from build123d import *

# Parameters (mm, degrees)
SKETCH037_R          = 1.6
SKETCH037_R_2        = 17
PAD006_DEPTH         = 3
SKETCH003_R          = 1.5
PAD007_DEPTH         = 22
SKETCH042_R          = 33.309059
POCKET028_DEPTH      = 18.95
SKETCH043_W          = 51.697506
SKETCH043_H          = 15.935999
POCKET029_DEPTH      = 28.801
POCKET029_DEPTH_BACK = 23.4566344398
SKETCH040_R          = 3
FILLET003_R          = 2
FILLET004_R          = 5
FILLET005_R          = 1


with BuildPart() as part:
    # Sketch037 → Pad006 (new body)
    with BuildSketch(Plane.XY.offset(8)):
        with BuildLine():
            Line((-25.5, 14.6837073124), (-25.5, -7.8162926876))
            Line((-5.3310209809, -19.2403151033), (-25.5, -7.8162926876))
            Line((11.1640063658, -23.3529873285), (-5.3310209809, -19.2403151033))
            ThreePointArc((11.1640063658, -23.3529873285), (13.7797833094, -22.9620568449), (15.3529873285, -20.8359936342))
            Line((19.8, -3), (15.3529873285, -20.8359936342))
            Line((19.8, 15.1005154776), (19.8, -3))
            ThreePointArc((19.8, 15.1005154776), (19.1301270189, 17.6005154776), (17.3, 19.4306424965))
            Line((2, 28.2641016151), (17.3, 19.4306424965))
            ThreePointArc((2, 28.2641016151), (0, 28.8), (-2, 28.2641016151))
            Line((-9.101080859, 23.5924155561), (-2, 28.2641016151))
            ThreePointArc((-15.8499401029, 19.751877), (-10.97303678, 19.0318958608), (-9.101080859, 23.5924155561))
            Line((-25.5, 14.6837073124), (-15.8499401029, 19.751877))
        make_face()
        with Locations((0, 24.8)):
            Circle(SKETCH037_R, mode=Mode.SUBTRACT)
        with Locations((12, -20)):
            Circle(SKETCH037_R, mode=Mode.SUBTRACT)
        with Locations((-21.5, 12.3)):
            Circle(SKETCH037_R, mode=Mode.SUBTRACT)
        Circle(SKETCH037_R_2, mode=Mode.SUBTRACT)
    extrude(amount=PAD006_DEPTH)

    # Sketch003 → Pad007 (join)
    with BuildSketch(Plane(origin=(-2.6, 10.8, 17), x_dir=(0.9021044144, 0.420580995, -0.0965362737), z_dir=(-0.1354559934, 0.4884043208, 0.8620399604))):
        with BuildLine():
            Line((-23.3696005315, -4.8773641565), (-13.621692219, 4.2127074032))
            ThreePointArc((-12.2576954989, 4.75), (-12.9906979524, 4.610835136), (-13.621692219, 4.2127074032))
            Line((-12.2576954989, 4.75), (10.0610339657, 4.75))
            ThreePointArc((10.780373766, 4.4446583705), (10.4517650942, 4.6705048535), (10.0610339657, 4.75))
            Line((10.780373766, 4.4446583705), (19.7793336026, -4.8740373329))
            ThreePointArc((21.0423045011, -8), (20.7146318466, -6.3142703296), (19.7793336026, -4.8740373329))
            Line((21.0423045011, -8), (21.0423045011, -15.35))
            ThreePointArc((20.0423045011, -16.35), (20.7494112823, -16.0571067812), (21.0423045011, -15.35))
            Line((20.0423045011, -16.35), (-8.9576954989, -16.35))
            Line((-8.9576954989, -16.35), (-21.8124305048, -12.0490416884))
            ThreePointArc((-23.3696005315, -4.8773641565), (-24.6301401013, -8.9059534041), (-21.8124305048, -12.0490416884))
        make_face()
        with Locations((16.5423045011, -8)):
            Circle(SKETCH003_R, mode=Mode.SUBTRACT)
        with Locations((-20.4576954989, -8)):
            Circle(SKETCH003_R, mode=Mode.SUBTRACT)
    extrude(amount=-PAD007_DEPTH)

    # Sketch042 → Pocket028 (cut, symmetric)
    with BuildSketch(Plane.XY.offset(8)):
        with Locations((0, 3.706026)):
            Circle(SKETCH042_R)
        with BuildLine():
            Line((-25.5, 14.6963702892), (-25.5, -7.8036297108))
            Line((-5.3310209809, -19.2403151033), (-25.5, -7.8036297108))
            Line((11.1640063658, -23.3529873285), (-5.3310209809, -19.2403151033))
            ThreePointArc((11.1640063658, -23.3529873285), (13.7797833094, -22.9620568449), (15.3529873285, -20.8359936342))
            Line((19.8, -3), (15.3529873285, -20.8359936342))
            Line((19.8, 15.1005154776), (19.8, -3))
            ThreePointArc((19.8, 15.1005154776), (19.1301270189, 17.6005154776), (17.3, 19.4306424965))
            Line((2, 28.2641016151), (17.3, 19.4306424965))
            ThreePointArc((2, 28.2641016151), (0, 28.8), (-2, 28.2641016151))
            Line((-25.5, 14.6963702892), (-2, 28.2641016151))
        make_face(mode=Mode.SUBTRACT)
    extrude(amount=POCKET028_DEPTH, both=True, mode=Mode.SUBTRACT)

    # Sketch043 → Pocket029 (cut, two sides)
    with BuildSketch(Plane.XZ) as pocket029_sk:
        with Locations((-1.406603, 0.0320005)):
            Rectangle(SKETCH043_W, SKETCH043_H)
    extrude(amount=-POCKET029_DEPTH, mode=Mode.SUBTRACT)
    extrude(pocket029_sk.sketch, amount=POCKET029_DEPTH_BACK, mode=Mode.SUBTRACT)

    # SubtractivePipe: sweep along a path in Sketch044
    with BuildLine(Plane(origin=(0, 0, 6), x_dir=(-0.3746065934, 0.9271838546, 0), z_dir=(0.9266190392, 0.3743783932, 0.0348994967))) as subtractivepipe_path:
        ThreePointArc((4.9840972168, 16.8364980654), (1.2784963095, 9.7214039712), (0, 1.801714))
    # Sketch040 → SubtractivePipe (sweep, cut)
    with BuildSketch(Plane(origin=(-2, 7.6, 8), x_dir=(0.8829475929, 0.4694715628, 0), z_dir=(0, 0, 1))):
        with Locations((-1.846382, -7.651343)):
            Circle(SKETCH040_R)
    sweep(path=subtractivepipe_path.line, mode=Mode.SUBTRACT)

    # Fillet003
    fillet003_edges = [part.edges().sort_by_distance(p)[0] for p in [
        (-9.101081, 23.592416, 9.5),
        (-15.84994, 19.751877, 9.5),
    ]]
    fillet(fillet003_edges, radius=FILLET003_R)

    # Fillet004
    fillet004_edges = [part.edges().sort_by_distance(p)[0] for p in [
        (-25.5, -7.80363, 9.5),
        (-25.5, 14.683707, 9.5),
    ]]
    fillet(fillet004_edges, radius=FILLET004_R)

    # Fillet005
    fillet005_edges = [part.edges().sort_by_distance(p)[0] for p in [
        (-4.660699, 2.190867, 21.553854),
    ]]
    fillet(fillet005_edges, radius=FILLET005_R)


solid = part.part
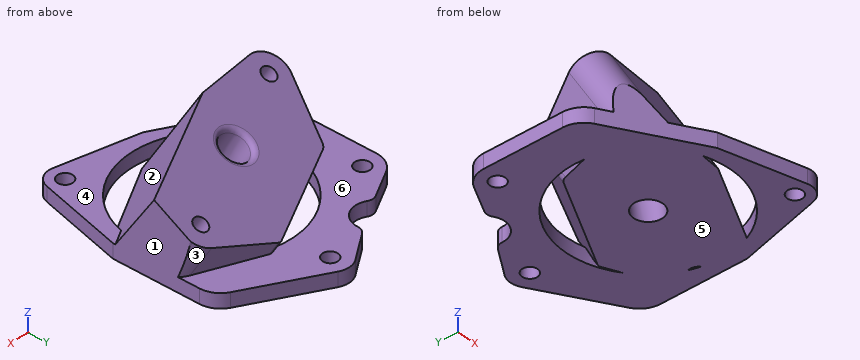
Could you check a few things on this model? Use its own coordinates, in mm. Face numbers are marked on the shaded views. A direction names the side the tool comes from. Give positions to 0.01 mm unless a question says otherwise; leave off trailing zeros. Loops run counter-clockwise (first coordinate to the right, second up) from the corner with the lowest first, then second, coordinate; pieces in that order, holes last. Notation, with made-up numbers: M 60.5,-9.5 L 92.5,-9.5 A25 ccw 92.5,2.5 Z; hole C -4.5,-7.5 d7. An arc over 180 degrees is marked long. Answer as a JSON object with one key per item and string values.
Q1. For P1, Ø3.5, axis at x = 17, y = 7, coming from the +Z side; P2, Ø23, axis at x = -0.5, y = -10.5, coming from the +Z side; P3, Ø2, axis at x = -19.5, z = 10.5, coming from the -Y side; P4, Ø1, axis at x = -12, z = 13, coming from the +Y side, each with a flat end and sliding along its axis, tell me the tip position at first contact or that it passes through.
Values found:
{"P1": "stops at z = 23.26", "P2": "stops at z = 26", "P3": "stops at y = -11.77", "P4": "stops at y = 9.79"}
Q2. If we mould it in two halves opening along Z, with no side actions, what happens to the marked faces 4, 5 and 6? For each: pulls with the +Z half, pulls with the -Z half, needs draft (parallel to the pull), parting line crosses it, or undercut.
Values found:
{"face 4": "pulls with the +Z half", "face 5": "pulls with the -Z half", "face 6": "undercut"}
Q3. For the marked faces 1, 2 and 3, which set-ups out of +Z, -Z, +X, -X, +Y, -Y let a thin tool reach every point of the face, with its end or its side?
Values found:
{"face 1": "+Z, -Z, +X, +Y, -Y", "face 2": "+Z", "face 3": "+X, +Y"}
Q4. Suppose I cut it at C-C, the plane x = 0. State how many separate pieces and enclosed holes the cut face has, plus the area to 3 significant figures.
Values found:
{"separate pieces": "5", "enclosed holes": "0", "area": "283 mm²"}
Q5. Suppose I cut it at A-A, the plane x = 12. List the corners of the cut face in (y, z) for me, plus the area to 3 significant figures.
Values found:
{"outline": "M -23.46,8 L -21.6,8 L -21.6,11 L -23.46,11 Z; M -18.4,8 L -12.04,8 L -12.04,11 L -18.4,11 Z; M -8.62,8 L 22.49,8 L 22.49,11 L 14.44,11 L 16.86,15.86 L 1.98,24.29 Z", "area": "302 mm²"}
Q6. If I drill on probe 1 along Y at (x, z) = (12, 8.65); probe 2 along Z at (x, y) = (-12.5, 9.5); probe 3 along Z at (x, y) = (2.5, 3.5), over which ranges is the centre line in solid material (lowest first)? Write a range as [from, to].
Values found:
{"probe 1": "y = [-23.46, -21.6], [-18.4, -12.04], [-8.19, 22.49]", "probe 2": "z = [13.61, 16.18]", "probe 3": "z = [8, 21.94]"}
Q7. Suppose I cut it at B-B, the plane y = -20. List the corners of the cut face in (x, z) for me.
Values found:
{"outline": "M -2.28,8 L 10.4,8 L 10.4,11 L -2.28,11 Z; M 13.6,8 L 15.56,8 L 15.56,11 L 13.6,11 Z"}
